Can you work these out from the model? Positions are in its coordinate system, mm. A direction names the side the tool comes from. Coordinates: 2 decimals unless noted, no trailing zeros. Order: outer loops, then holes, each group sorted by start corner. A loop starts at its lowest first (then second) coordinate and runs counter-clockwise, first axis right, second up. Notation, with made-up numbers: (36.5, -22) - (91.5, -22) arc R24 ccw to (91.5, -3) - close; hole circle Ø1 at (4.25, -27.75). An arc over 180 degrees is marked (long way). Return JSON: item names as keys, results as strings. Group by question number.
1) If I drill on line 1 along Z through (x, y) = (0, 1.05); line 2 along Z through (x, y) = (12, 1.75); line 3 along X through (y, z) = (1, -9), over which ranges is the centre line in solid material (lowest first)?
2) Imagine slicing it at D-D (x = 39). Write out the boundary of the cut face in (y, z).
3) Imagine slicing it at B-B (z = 34.5). Write out the boundary of the cut face in (x, y).
4) If we mould it in two halves opening along X, with no side actions, what happens to faces 4 (the face through (-50.09, 1.03, 15.77)), 5 (the face through (1, 6.35, -12)), 6 (the face through (57.095, 3.219, 2.513))? For each: pulls with the +X half, pulls with the -X half, needs draft (parallel to the pull), parting line crosses it, or undercut.
5) Imagine slicing it at A-A (x = 0). Write out the boundary of the cut face in (y, z), and give its area (3 significant figures).
6) Which directions (+Z, -Z, +X, -X, +Y, -Y) give clear straight access to the entire face, cutting with the end or side of a thin tool? Please do faces 1 (the face through (-33.2, 2.032, -40.9)), 2 (the face through (-42.79, 4.74, -0.48)), 3 (the face through (-47, 0, 30)).
7) Imagine slicing it at C-C (y = 5.25). Give the number of separate pieces and of enclosed holes in the cut face, and give its area (3 significant figures).
8) For pin 1 Ø8 at (x, z) = (4, -1.5) entering from -Y; pin 2 Ø3 at (x, z) = (-41.275, 0) entering from +Y; pin 3 Ø1.5 at (y, z) = (3, 45.5) entering from -X, each with a flat end and sliding along its axis, tell me the tip position at first contact or that it passes through.
```python
from build123d import *

# Parameters (mm, degrees)
F_1_8_0_125_DIAMETER_HOLE1_D     = 3.175
F_1_8_0_125_DIAMETER_HOLE1_DEPTH = 3.175
F_1_8_0_125_DIAMETER_HOLE1_TIP   = 0.953866233


with BuildPart() as part:
    # Sketch1 → Revolve1 (revolve)
    with BuildSketch(Plane.XY):
        Polygon((-6.35, 0), (-52.5145, 0), (-52.5145, 2.032), (-55.5625, 2.032), (-55.5625, 0), (-57.15, 0), (-57.15, 6.35), (-6.35, 6.35), align=None)
    revolve(axis=Axis((0, 0, 0), (0, 1, 0)))

    # 1/8 (0.125) Diameter Hole1
    with Locations(Plane(origin=(0, 6.35, 0), x_dir=(1, 0, 0), z_dir=(0, 1, 0))):
        with Locations((-41.275, 0)):
            Hole(F_1_8_0_125_DIAMETER_HOLE1_D / 2, depth=F_1_8_0_125_DIAMETER_HOLE1_DEPTH)
            with Locations((0, 0, -(F_1_8_0_125_DIAMETER_HOLE1_DEPTH + F_1_8_0_125_DIAMETER_HOLE1_TIP / 2))):  # 118° drill point
                Cone(0, F_1_8_0_125_DIAMETER_HOLE1_D / 2, F_1_8_0_125_DIAMETER_HOLE1_TIP, mode=Mode.SUBTRACT)


solid = part.part
```
Calculated:
{
 "1": {"line 1": "-57.15 to -55.56, -52.51 to -6.35, 6.35 to 52.51, 55.56 to 57.15", "line 2": "-55.88 to -54.25, -51.13 to 51.13, 54.25 to 55.88", "line 3": "-56.44 to -54.83, -51.74 to 51.74, 54.83 to 56.44"},
 "2": {"outline": "(0, -41.77) - (6.35, -41.77) - (6.35, 41.77) - (0, 41.77) - (0, 39.58) - (2.03, 39.58) - (2.03, 35.17) - (0, 35.17) - (0, -35.17) - (2.03, -35.17) - (2.03, -39.58) - (0, -39.58) - close"},
 "3": {"outline": "(-45.56, 0) - (-43.55, 0) - (-43.55, 2.03) - (-39.59, 2.03) - (-39.59, 0) - (39.59, 0) - (39.59, 2.03) - (43.55, 2.03) - (43.55, 0) - (45.56, 0) - (45.56, 6.35) - (-45.56, 6.35) - close"},
 "4": {"face 4": "undercut", "face 5": "needs draft", "face 6": "parting line crosses it"},
 "5": {"outline": "(0, -57.15) - (6.35, -57.15) - (6.35, -6.35) - (0, -6.35) - (0, -52.51) - (2.03, -52.51) - (2.03, -55.56) - (0, -55.56) - close; (0, 6.35) - (6.35, 6.35) - (6.35, 57.15) - (0, 57.15) - (0, 55.56) - (2.03, 55.56) - (2.03, 52.51) - (0, 52.51) - close", "area": "633 mm2"},
 "6": {"face 1": "-Y", "face 2": "+Y", "face 3": "+Z, -Z, +X, -X, -Y"},
 "7": {"separate pieces": "1", "enclosed holes": "2", "area": "10,100 mm2"},
 "8": {"pin 1": "y = 0", "pin 2": "y = 3.12", "pin 3": "x = -35.55"}
}
